Geometry: final body of the model. Coordinates: model frame, mm. Face numbers are marked on the shaded views. A direction names the side the tool comes from. Coordinates: 2 decimals unless noted, no trailing zeros. Order: outer loops, then holes, each group sorted by start corner. A loop starts at its lowest first (then second) coordinate and runs counter-clockwise, first axis right, second up. Notation, with made-up numbers: (55, 43.5) - (72, 43.5) arc R25 ccw to (72, 61.5) - close; hole circle Ø6 at (-32.75, -38.75). An arc over 180 degrees is marked (long way). Use one line per item in the form item = value. Start each with the question number.
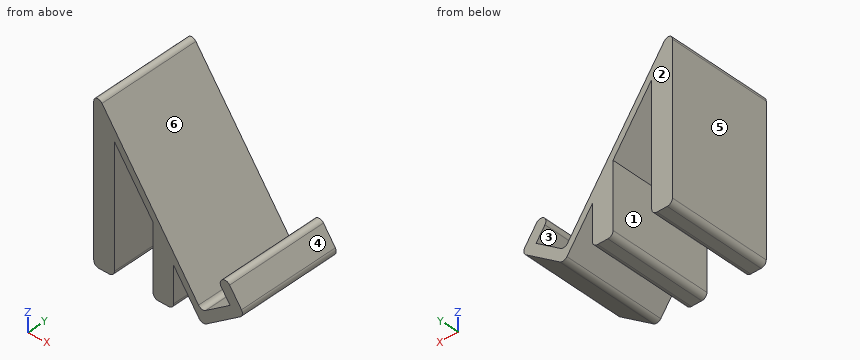
```python
from build123d import *

# Parameters (mm, degrees)
F1_DEPTH    = 101.6
F3_DEPTH    = 6.35
F5_DEPTH    = 44.45
F6_W        = 10.16
F6_H        = 101.6
F7_DEPTH    = 20.32
F8_T1_DEPTH = 101.6
F8_T3_DEPTH = 127
F8_T5_DEPTH = 114.822403084
F10_W       = 251.0453239083
F10_H       = 203.9344906807
F11_DEPTH   = 160.782


# Not quite as in the source:
# - a fillet or chamfer that OpenCascade refuses, or shapes differently, is made with other operations: its cross-section is extruded or revolved along the edge and cut away or added


with BuildPart() as f1:
    # F0 (on Front) → F1 (new body)
    with BuildSketch(Plane.XZ):
        Polygon((57.3137016242, -18.4824153282), (36.9937016242, 10.5375521688), (36.9937016242, -58.4300412773), (57.3137016242, -58.4300412773), align=None)
    extrude(amount=F1_DEPTH)



with BuildPart() as f1b:
    # F0 (on Front) → F1, piece 2 (new body)
    with BuildSketch(Plane.XZ):
        Polygon((-1.1062983758, 64.9499912257), (-21.4262983758, 93.9699587227), (-21.4262983758, -58.4300412773), (-1.1062983758, -58.4300412773), align=None)
    extrude(amount=F1_DEPTH)


with BuildPart() as f1_1:
    add(f1.part)

    add(f1b.part)  # F3 merges F1b
    # F2 (on face) → F3 (join)
    with BuildSketch(Plane(origin=(29.774176385, 0, 20.8481027487), x_dir=(0, 1, 0), z_dir=(0.8191520443, 0, 0.5735764364))):
        Polygon((-101.6, 89.265303656), (-101.6, -96.780755544), (0, -96.780755544), (0, 38.465303656), (0, 89.265303656), align=None)
    extrude(amount=F3_DEPTH)

    # F4 (on face) → F5 (join)
    with BuildSketch(Plane(origin=(34.9757918662, 0, 24.4903131196), x_dir=(0, 1, 0), z_dir=(0.8191520443, 0, 0.5735764364))):
        Polygon((-101.6, -86.620755544), (-101.6, -96.780755544), (0, -96.780755544), (0, -86.620755544), (-12.7, -86.620755544), (-88.9, -86.620755544), align=None)
    extrude(amount=F5_DEPTH)

    # F6 (on face) → F7 (join)
    with BuildSketch(Plane(origin=(49.6836242789, 0, -70.9555689817), x_dir=(0.8191520443, 0, 0.5735764364), z_dir=(-0.5735764364, 0, 0.8191520443))):
        with Locations((82.0675579321, -50.8)):
            Rectangle(F6_W, F6_H)
    extrude(amount=F7_DEPTH)

    # F8: fillet of radius 5.08 on 11 edges, made by hand

    # F8_s2 → F8_t1 (join)
    with BuildSketch(Plane.XZ):
        with BuildLine():
            ThreePointArc((81.7456478485, -42.3039634771), (85.0248074909, -44.3930185658), (88.8207085301, -43.5514875655))
            Line((88.8207085301, -43.5514875655), (84.6594161452, -46.4652558621))
            Line((84.6594161452, -46.4652558621), (81.7456478485, -42.3039634771))
        make_face()
    extrude(amount=F8_T1_DEPTH)

    # F8_s4 → F8_t3 (cut)
    with BuildSketch(Plane.XZ.offset(-12.7)):
        with BuildLine():
            ThreePointArc((112.3294196238, -8.4859061114), (109.0502599814, -6.3968510227), (105.2543589422, -7.238382023))
            Line((105.2543589422, -7.238382023), (109.4156513272, -4.3246137264))
            Line((109.4156513272, -4.3246137264), (112.3294196238, -8.4859061114))
        make_face()
        with BuildLine():
            ThreePointArc((122.7369687221, -32.206136333), (124.8260238108, -28.9269766905), (123.9844928105, -25.1310756513))
            Line((123.9844928105, -25.1310756513), (126.8982611071, -29.2923680363))
            Line((126.8982611071, -29.2923680363), (122.7369687221, -32.206136333))
        make_face()
        with BuildLine():
            ThreePointArc((105.2543589422, -7.238382023), (103.1653038535, -10.5175416655), (104.0068348538, -14.3134427047))
            Line((104.0068348538, -14.3134427047), (101.0930665572, -10.1521503197))
            Line((101.0930665572, -10.1521503197), (105.2543589422, -7.238382023))
        make_face()
        with BuildLine():
            ThreePointArc((-13.3109145979, 93.4508767085), (-16.5900742404, 95.5399317971), (-20.3859752796, 94.6984007968))
            Line((-20.3859752796, 94.6984007968), (-16.2246828946, 97.6121690935))
            Line((-16.2246828946, 97.6121690935), (-13.3109145979, 93.4508767085))
        make_face()
        with BuildLine():
            ThreePointArc((82.3715689606, -54.2687586179), (85.650728603, -56.3578137066), (89.4466296422, -55.5162827063))
            Line((89.4466296422, -55.5162827063), (85.2853372573, -58.4300510029))
            Line((85.2853372573, -58.4300510029), (82.3715689606, -54.2687586179))
        make_face()
        with BuildLine():
            ThreePointArc((-16.3462983758, -58.4300412773), (-19.9384008243, -56.9421437258), (-21.4262983758, -53.3500412773))
            Line((-21.4262983758, -53.3500412773), (-21.4262983758, -58.4300412773))
            Line((-21.4262983758, -58.4300412773), (-16.3462983758, -58.4300412773))
        make_face()
        with BuildLine():
            ThreePointArc((-1.1062983758, -53.3500412773), (-2.5941959274, -56.9421437258), (-6.1862983758, -58.4300412773))
            Line((-6.1862983758, -58.4300412773), (-1.1062983758, -58.4300412773))
            Line((-1.1062983758, -58.4300412773), (-1.1062983758, -53.3500412773))
        make_face()
        with BuildLine():
            ThreePointArc((36.9937016242, -53.3500412773), (38.4815991757, -56.9421437258), (42.0737016242, -58.4300412773))
            Line((42.0737016242, -58.4300412773), (36.9937016242, -58.4300412773))
            Line((36.9937016242, -58.4300412773), (36.9937016242, -53.3500412773))
        make_face()
        with BuildLine():
            ThreePointArc((52.2337016242, -58.4300412773), (55.8258040726, -56.9421437258), (57.3137016242, -53.3500412773))
            Line((57.3137016242, -53.3500412773), (57.3137016242, -58.4300412773))
            Line((57.3137016242, -58.4300412773), (52.2337016242, -58.4300412773))
        make_face()
    extrude(amount=F8_T3_DEPTH, mode=Mode.SUBTRACT)

    # F8_s6 → F8_t5 (cut)
    with BuildSketch(Plane.XZ.offset(-6.611201542)):
        with BuildLine():
            ThreePointArc((-21.4262983758, 91.3254781059), (-20.8523134084, 93.6711610611), (-19.2600666725, 95.4867704908))
            Line((-19.2600666725, 95.4867704908), (-21.4262983758, 93.9699587227))
            Line((-21.4262983758, 93.9699587227), (-21.4262983758, 91.3254781059))
        make_face()
    extrude(amount=F8_T5_DEPTH, mode=Mode.SUBTRACT)


with BuildPart() as f9_1:
    # F9: copy of F1
    add(f1_1.part.moved(Location((0, 169.418, 0))))

    # F10 (on face) → F11 (cut)
    with BuildSketch(Plane.XZ.offset(-67.818)):
        with Locations((60.7606135309, 16.4267346263)):
            Rectangle(F10_W, F10_H)
    extrude(amount=-F11_DEPTH, mode=Mode.SUBTRACT)


solid = f1_1.part
```
(1) Draft query along X for the marked faces 4, 5 and 6. Return one class per face: released by +X, released by -X, zero draft, split by the parting line, or undercut.
(2) Cut plane A-A on z = -10.5. Return the cut outline in (x, y), plus the area to 3 significant figures.
(3) Material intervals for L1, parallel to X at y = -71, z = 27; L2, parallel to X at y = -68, z = 32; L3, parallel to X at y = -56.5, z = -24, sorted ascending. Write a range as from..to.
(4) Contact query for flat-ended pins moving along their axis: pin 1 Ø2 at (x, y) = (107, -20) entering from -Z; pin 2 Ø1.5 at (y, z) = (-50.5, -7.5) entering from +X. Output: stop coordinate, or through.
(5) Cut plane D-D on x = 32. Return the cut outline in (y, z).
(6) Cut plane C-C on z = 15. Return the cut outline in (x, y), plus the area to 3 significant figures.
(7) Set-up query: the marked faces 1, 2 and 3. Return all of +Z, -Z, +X, -X, +Y, -Y with unobstructed straight access to the full face (end or side cutting, diameter ignored); none if empty.
Check sheet entries:
q1.face_4 = released by +X
q1.face_5 = released by -X
q1.face_6 = undercut
q2.outline = (-21.43, -101.6) - (-1.11, -101.6) - (-1.11, 0) - (-21.43, 0) - close; (36.99, -101.6) - (59.48, -101.6) - (59.48, 0) - (36.99, 0) - close; (103.17, -101.6) - (113.74, -101.6) - (113.74, 0) - (103.17, 0) - close
q2.area = 5,420 mm^2
q3.L1 = -21.43..-1.11, 25.47..33.22
q3.L2 = -21.43..-1.11, 21.97..29.72
q3.L3 = -21.43..-1.11, 36.99..57.31, 61.18..68.93, 110.79..123.19
q4.pin_1 = -43.93
q4.pin_2 = 112.15
q5.outline = (-101.6, 17.67) - (0, 17.67) - (0, 28.74) - (-101.6, 28.74) - close
q6.outline = (-21.43, -101.6) - (-1.11, -101.6) - (-1.11, 0) - (-21.43, 0) - close; (33.87, -101.6) - (41.62, -101.6) - (41.62, 0) - (33.87, 0) - close
q6.area = 2,850 mm^2
q7.face_1 = -Z, +Y, -Y
q7.face_2 = +Z, -Z, +X, -X, +Y
q7.face_3 = +Y, -Y
